from build123d import *

# Parameters (mm, degrees)
REVOLUCI_N1_ANGLE       = 90
SALIENTE_EXTRUIR1_START = -10
SALIENTE_EXTRUIR1_DEPTH = 10
REDONDEO1_R             = 6
CROQUIS5_R              = 3
CORTAR_EXTRUIR1_DEPTH   = 156.393050206
REDONDEO2_R             = 5
CORTAR_EXTRUIR3_DEPTH   = 157.140962122
CORTAR_EXTRUIR4_DEPTH   = 152.400132213


with BuildPart() as part:
    # Croquis3 → Revolución1 (revolve)
    with BuildSketch(Plane(origin=(0, 0, 0), x_dir=(0, 0, -1), z_dir=(1, 0, 0))):
        with BuildLine():
            Line((25.795554958, 0), (25.795554958, 5.555717972))
            Line((25.795554958, 5.555717972), (48, 60))
            Line((48, 60), (48, 91))
            Line((48, 91), (54, 91))
            Line((54, 91), (54, 60))
            Line((54, 60), (30.939888656, 3.457663399))
            ThreePointArc((30.939888656, 3.457663399), (28.894732485, 0.944741845), (25.795554958, 0))
        make_face()
    revolve(axis=Axis((0, 0, 0), (0, 1, 0)), revolution_arc=REVOLUCI_N1_ANGLE)

    # Croquis4 → Saliente-Extruir1 (add)
    with BuildSketch(Plane(origin=(0, 91, 0), x_dir=(1, 0, 0), z_dir=(0, 1, 0)).offset(SALIENTE_EXTRUIR1_START)):
        with BuildLine():
            Line((-85.559920524, 36.062445841), (-74.953318806, 46.669047558))
            Line((-74.953318806, 46.669047558), (-49.610431326, 21.326160078))
            ThreePointArc((-49.610431326, 21.326160078), (-52.411957015, 12.999490829), (-53.826220039, 4.328745356))
            Line((-53.826220039, 4.328745356), (-85.559920524, 36.062445841))
        make_face()
        with BuildLine():
            Line((-46.669047558, 74.953318806), (-21.326160078, 49.610431326))
            ThreePointArc((-21.326160078, 49.610431326), (-12.999490829, 52.411957015), (-4.328745356, 53.826220039))
            Line((-4.328745356, 53.826220039), (-36.062445841, 85.559920524))
            Line((-36.062445841, 85.559920524), (-46.669047558, 74.953318806))
        make_face()
    extrude(amount=SALIENTE_EXTRUIR1_DEPTH)

    # Redondeo1
    redondeo1_edges = [part.edges().sort_by_distance(p)[0] for p in [
        (-52.411957015, 81, -12.999490829),
        (-12.999490829, 81, -52.411957015),
    ]]
    fillet(redondeo1_edges, radius=REDONDEO1_R)

    # Croquis5 → Cortar-Extruir1 (cut, through all)
    with BuildSketch(Plane(origin=(-24.748737342, 0, 24.748737342), x_dir=(0.707106781186549, 0, 0.707106781186546), z_dir=(-0.707106781186546, 0, 0.707106781186549))):
        with Locations((-59, 86)):
            Circle(CROQUIS5_R)
        with Locations((-78, 86)):
            Circle(CROQUIS5_R)
    extrude(amount=-CORTAR_EXTRUIR1_DEPTH, mode=Mode.SUBTRACT)

    # Redondeo2
    redondeo2_edges = [part.edges().sort_by_distance(p)[0] for p in [
        (-80.256619665, 81, -41.365746699),
        (-41.365746699, 81, -80.256619665),
        (-80.256619665, 91, -41.365746699),
        (-41.365746699, 91, -80.256619665),
    ]]
    fillet(redondeo2_edges, radius=REDONDEO2_R - 0.0001)  # a hair under: the kernel refuses the full size

    # Croquis14 → Cortar-Extruir3 (cut, through all)
    with BuildSketch(Plane(origin=(27, 0, -27), x_dir=(-0.7071067811865492, 0, -0.7071067811865458), z_dir=(0.7071067811865458, 0, -0.7071067811865492))):
        with BuildLine():
            Line((34.445016975, 91), (33.941125497, 91))
            Line((33.941125497, 91), (33.941125497, 86))
            ThreePointArc((33.941125497, 86), (34.067416606, 88.512663259), (34.445016975, 91))
        make_face()
    extrude(amount=-CORTAR_EXTRUIR3_DEPTH, mode=Mode.SUBTRACT)

    # Croquis17 → Cortar-Extruir4 (cut, through all)
    with BuildSketch(Plane(origin=(0, 91, 0), x_dir=(1, 0, 0), z_dir=(0, 1, 0))):
        with BuildLine():
            Line((-4.328745356, 53.826220039), (0, 48.712610162))
            Line((0, 48.712610162), (0, 54))
            ThreePointArc((0, 54), (-2.1661161, 53.956537519), (-4.328745356, 53.826220039))
        make_face()
        with BuildLine():
            Line((-53.826220039, 4.328745356), (-48.712610162, 0))
            Line((-48.712610162, 0), (-54, 0))
            ThreePointArc((-54, 0), (-53.956537519, 2.1661161), (-53.826220039, 4.328745356))
        make_face()
    extrude(amount=-CORTAR_EXTRUIR4_DEPTH, mode=Mode.SUBTRACT)


solid = part.part
Check sheet for the modelled part. Datum: model origin and axes. Units: mm. A direction names the side the tool comes from. Give positions to 0.01 mm unless a question says otherwise; leave off trailing zeros. Order: outer loops, then holes, each group sorted by start corner. A loop starts at its lowest first (then second) coordinate and runs counter-clockwise, first axis right, second up. Notation, with made-up numbers: (-36.5, -6.5) - (-0.5, -6.5) arc R24 ccw to (-0.5, 18.5) - close; hole circle Ø6 at (6.25, 73). An arc over 180 degrees is marked (long way). Answer as CSV lines item,"result".
1. Section check C-C (y = 18.5). Record the boundary of the cut face in (x, z).
Result sheet:
outline,"(-37.07, 0) arc R37.07 ccw to (0, -37.07) - (0, -31.07) arc R31.07 cw to (-31.07, 0) - close"
2. Scan lines: probe 1 along Y at (x, z) = (-28, -59); probe 2 along Y at (x, z) = (-58.5, -14); probe 3 along Z at (x, y) = (-23, 78.5). Record each from-to range of solid material in increasing order. Write a range as from..to.
Result sheet:
probe 1,"81..84.37, 87.63..91"
probe 2,"81..91"
probe 3,"-48.86..-42.13"
3. Tool access check on faces 1 (the face through (-68, 81, -27)), 2 (the face through (-69.5, 84.7, -20)), 3 (the face through (-37.805, 71.839, -38.559)). Record the directions out of +Z, -Z, +X, -X, +Y, -Y that give a thin tool (end or side, any length) a straight path to the whole face; none if there is none.
Result sheet:
face 1,"-Z, -X, -Y"
face 2,"+Z, -X, +Y, -Y"
face 3,"-Y"
4. Section check B-B (z = -24). State how many separate pieces and enclosed holes the cut face has, then the cut area to 3 significant figures.
Result sheet:
separate pieces,"2"
enclosed holes,"1"
area,"864 mm²"
5. Section check A-A (y = 62.5). Record the boundary of the cut face in (x, z), then the cut area to 3 significant figures.
Result sheet:
outline,"(-53.83, -4.33) arc R54 ccw to (-4.33, -53.83) - (0, -48.71) - (0, -48) arc R48 cw to (-48, 0) - (-48.71, 0) - close"
area,"458 mm²"
6. Section check D-D (y = 28). Record the boundary of the cut face in (x, z), then the cut area to 3 significant figures.
Result sheet:
outline,"(-40.95, 0) arc R40.95 ccw to (0, -40.95) - (0, -34.95) arc R34.95 cw to (-34.95, 0) - close"
area,"358 mm²"
7. Go/stop test with flat-tipped pins: P1, Ø1, axis at x = -27.5, y = 81, coming from the +Z side; P2, Ø14, axis at x = -23, z = -65.5, coming from the -Y side; P3, Ø5, axis at x = -19, y = 27.5, coming from the -Z side. Record where each tip stops, or that it passes through.
Result sheet:
P1,"z = -38.99"
P2,"y = 81"
P3,"z = -37.72"
8. Mould release check, pull along Z, two halves, no side actions. Record for faces 4 (the face through (-36.24, 83.07, -74.99)), 5 (the face through (-25.91, 33.16, -26.49)), 6 (the face through (0, 32, -39)), 7 (the face through (-40.38, 89.57, -79.12)): released by +Z, released by -Z, zero draft, split by the parting line, or undercut.
Result sheet:
face 4,"undercut"
face 5,"released by +Z"
face 6,"zero draft"
face 7,"released by -Z"
